```python
from build123d import *

# Parameters (mm, degrees)
BOSS_EXTRUDE1_DEPTH             = 400
CUT_EXTRUDE1_DEPTH              = 401.906229685
CUT_EXTRUDE1_DEPTH_BACK         = 401.906229685
SKETCH2_R                       = 8.3125
CUT_EXTRUDE2_DEPTH              = 401.906229685
CUT_EXTRUDE2_DEPTH_BACK         = 401.906229685
SKETCH3_R                       = 3.38
CUT_EXTRUDE3_DEPTH              = 401.906229685
CUT_EXTRUDE3_DEPTH_BACK         = 401.906229685
SKETCH4_R                       = 3.38
BROOM_MOUNTING_HOLES_DEPTH      = 401.906229685
BROOM_MOUNTING_HOLES_DEPTH_BACK = 401.906229685
SKETCH6_R                       = 6.725


with BuildPart() as part:
    # Sketch1 → Boss-Extrude1 (new body)
    with BuildSketch(Plane.XY):
        with BuildLine():
            Line((-14.05, 19.05), (14.05, 19.05))
            ThreePointArc((14.05, 19.05), (17.585533906, 17.585533906), (19.05, 14.05))
            Line((19.05, 14.05), (19.05, -14.05))
            ThreePointArc((19.05, -14.05), (17.585533906, -17.585533906), (14.05, -19.05))
            Line((14.05, -19.05), (-14.05, -19.05))
            ThreePointArc((-14.05, -19.05), (-17.585533906, -17.585533906), (-19.05, -14.05))
            Line((-19.05, -14.05), (-19.05, 14.05))
            ThreePointArc((-19.05, 14.05), (-17.585533906, 17.585533906), (-14.05, 19.05))
        make_face()
        with BuildLine():
            Line((-15.875, 14.05), (-15.875, -14.05))
            ThreePointArc((-15.875, -14.05), (-15.340469876, -15.340469876), (-14.05, -15.875))
            Line((-14.05, -15.875), (14.05, -15.875))
            ThreePointArc((14.05, -15.875), (15.340469876, -15.340469876), (15.875, -14.05))
            Line((15.875, -14.05), (15.875, 14.05))
            ThreePointArc((15.875, 14.05), (15.340469876, 15.340469876), (14.05, 15.875))
            Line((14.05, 15.875), (-14.05, 15.875))
            ThreePointArc((-14.05, 15.875), (-15.340469876, 15.340469876), (-15.875, 14.05))
        make_face(mode=Mode.SUBTRACT)
    extrude(amount=BOSS_EXTRUDE1_DEPTH)

    # Sketch2 → Cut-Extrude1 (cut, two sides: drawn at the far end of the back side and taken through both)
    with BuildSketch(Plane(origin=(0, 0, 0), x_dir=(0, 0, -1), z_dir=(1, 0, 0)).offset(-CUT_EXTRUDE1_DEPTH_BACK)):
        with Locations((-375, 0)):
            Circle(SKETCH2_R)
        with Locations((-25, 0)):
            Circle(SKETCH2_R)
    extrude(amount=CUT_EXTRUDE1_DEPTH + CUT_EXTRUDE1_DEPTH_BACK, mode=Mode.SUBTRACT)

    # Sketch3 → Cut-Extrude2 (cut, two sides: drawn at the far end of the back side and taken through both)
    with BuildSketch(Plane(origin=(0, 0, 0), x_dir=(1, 0, 0), z_dir=(0, 1, 0)).offset(-CUT_EXTRUDE2_DEPTH_BACK)):
        with Locations(Location((0, -325, 0), (0, 0, 90))):
            Circle(SKETCH3_R)
        with Locations(Location((0, -75, 0), (0, 0, 90))):
            Circle(SKETCH3_R)
    extrude(amount=CUT_EXTRUDE2_DEPTH + CUT_EXTRUDE2_DEPTH_BACK, mode=Mode.SUBTRACT)

    # Sketch4 → Cut-Extrude3 (cut, two sides: drawn at the far end of the back side and taken through both)
    with BuildSketch(Plane(origin=(0, 0, 0), x_dir=(0, 0, -1), z_dir=(1, 0, 0)).offset(-CUT_EXTRUDE3_DEPTH_BACK)):
        with Locations((-200, 0)):
            Circle(SKETCH4_R)
    extrude(amount=CUT_EXTRUDE3_DEPTH + CUT_EXTRUDE3_DEPTH_BACK, mode=Mode.SUBTRACT)

    # Sketch6 → Broom Mounting Holes (cut, two sides: drawn at the far end of the back side and taken through both)
    with BuildSketch(Plane(origin=(0, 0, 0), x_dir=(1, 0, 0), z_dir=(0, 1, 0)).offset(-BROOM_MOUNTING_HOLES_DEPTH_BACK)):
        with Locations(Location((0, -112.5, 0), (0, 0, 270))):
            Circle(SKETCH6_R)
        with Locations(Location((0, -287.5, 0), (0, 0, 270))):
            Circle(SKETCH6_R)
    extrude(amount=BROOM_MOUNTING_HOLES_DEPTH + BROOM_MOUNTING_HOLES_DEPTH_BACK, mode=Mode.SUBTRACT)


solid = part.part
```
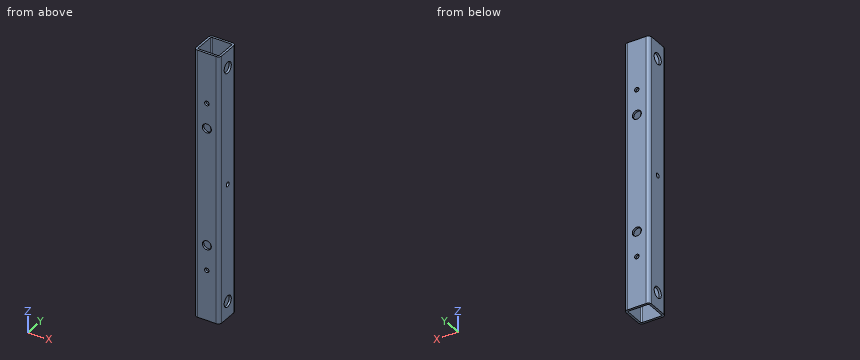
Geometry check sheet. Reference: the model listing, model coordinates, mm. Coordinates: 2 decimals unless noted, no trailing zeros. Loops run counter-clockwise (first coordinate to the right, second up) from the corner with the lowest first, then second, coordinate; pieces in that order, holes last.
Item 1: Sectioned sample at A-A, the plane z = 75. Record the boundary of the cut face in (x, y) (3 decimals).
Item 2: Go/stop test with a flat-tipped pin: pin 1 Ø6 at (x, z) = (0, 75) entering from -Y. Record where the tip stops, or that it passes through.
Item 3: Sectioned sample at C-C, the plane y = 0. Count the separate pieces of the cut face and the enclosed holes in it, then the cut area to 3 significant figures.
Item 4: Sectioned sample at B-B, the plane z = 210. Record the boundary of the cut face in (x, y) (3 decimals), then the cut area to 3 significant figures.
Item 5: Thickness scan on line 1 (Z direction, x = 17.5, y = 0); line 2 (Z direction, x = 17.5, y = -7); line 3 (Y direction, x = 2.5, z = 359) (3 decimals). Record the ranges inside material, lowest first.
Check result:
1. outline: (-19.05, -14.05) arc R5 ccw to (-14.05, -19.05) - (-3.38, -19.05) - (-3.38, -15.875) - (-14.05, -15.875) arc R1.825 cw to (-15.875, -14.05) - (-15.875, 14.05) arc R1.825 cw to (-14.05, 15.875) - (-3.38, 15.875) - (-3.38, 19.05) - (-14.05, 19.05) arc R5 ccw to (-19.05, 14.05) - close; (3.38, -19.05) - (14.05, -19.05) arc R5 ccw to (19.05, -14.05) - (19.05, 14.05) arc R5 ccw to (14.05, 19.05) - (3.38, 19.05) - (3.38, 15.875) - (14.05, 15.875) arc R1.825 cw to (15.875, 14.05) - (15.875, -14.05) arc R1.825 cw to (14.05, -15.875) - (3.38, -15.875) - close
2. pin 1: passes through
3. separate pieces: 8
3. enclosed holes: 0
3. area: 2,290 mm2
4. outline: (-19.05, -14.05) arc R5 ccw to (-14.05, -19.05) - (14.05, -19.05) arc R5 ccw to (19.05, -14.05) - (19.05, 14.05) arc R5 ccw to (14.05, 19.05) - (-14.05, 19.05) arc R5 ccw to (-19.05, 14.05) - close; hole (-15.875, -14.05) arc R1.825 ccw to (-14.05, -15.875) - (14.05, -15.875) arc R1.825 ccw to (15.875, -14.05) - (15.875, 14.05) arc R1.825 ccw to (14.05, 15.875) - (-14.05, 15.875) arc R1.825 ccw to (-15.875, 14.05) - close
4. area: 425 mm2
5. line 1: z = 0 to 16.69, 33.31 to 196.62, 203.38 to 366.69, 383.31 to 400
5. line 2: z = 0 to 20.52, 29.48 to 370.52, 379.48 to 400
5. line 3: y = -19.05 to -15.875, 15.875 to 19.05
